Autodesk Inventor part; units mm, degrees
ref_plane "YZ Plane" through (0, 0, 0) normal (1, 0, 0) x (0, 1, 0)
ref_plane "XZ Plane" through (0, 0, 0) normal (0, 1, 0) x (-1, 0, 0)
ref_plane "XY Plane" through (0, 0, 0) normal (0, 0, 1) x (1, 0, 0)
sketch "Sketch1" plane through (0, 0, 0) normal (0, 0, 1) x (1, 0, 0)
  line L0 (0, 0) -> (12.7, 0)
  line L1 (12.7, 0) -> (12.7, 12.7)
  line L2 (12.7, 12.7) -> (0, 12.7)
  line L3 (0, 12.7) -> (0, 0)
  circle A0 centre (6.35, 6.35) radius 5.08
  dimension "d0" = 12.7
  dimension "d1" = 12.7
  dimension "d2" = 10.16
extrude "Extrusion1" add sketch "Sketch1" along normal blind 3.175
extrude "Extrusion2" add sketch "Sketch1" along normal blind 12.7 contours A0
sketch "Sketch2" plane through (6.35, 6.35, 12.7) normal (0, 0, 1) x (1, 0, 0)
  circle A0 centre (0, 0) radius 2.2451
  point P0 (-6.35, -6.35)
extrude "Extrusion3" cut sketch "Sketch2" against normal blind 25.4
properties part number "TestPart1"
The listing builds one solid part. Answer for the finished solid, in the listing's coordinates (mm). A direction names the side the tool comes from. Give positions to 0.01 mm unless a question says otherwise; leave off trailing zeros. Order: outer loops, then holes, each group sorted by start corner. A loop starts at its lowest first (then second) coordinate and runs counter-clockwise, first axis right, second up. Notation, with made-up numbers: (21.25, 8.5) - (66.25, 8.5) arc R8 cw to (66.25, 12.5) - close; hole circle Ø5 at (79.5, 88.5). An arc over 180 degrees is marked (long way). Answer as CSV lines item,"result".
Q1. A cutting plane is placed at C-C, the plane z = 2.5. Determine the outline of the cut face in (x, y), and give its area (3 significant figures).
Answer key:
outline,"(0, 0) - (12.7, 0) - (12.7, 12.7) - (0, 12.7) - close; hole circle Ø4.49 at (6.35, 6.35)"
area,"145 mm^2"
Q2. A cutting plane is placed at A-A, the plane y = 6.35. Determine the outline of the cut face in (x, z) (3 decimals).
Answer key:
outline,"(0, 0) - (4.105, 0) - (4.105, 12.7) - (1.27, 12.7) - (1.27, 3.175) - (0, 3.175) - close; (8.595, 0) - (12.7, 0) - (12.7, 3.175) - (11.43, 3.175) - (11.43, 12.7) - (8.595, 12.7) - close"
Q3. Straight lines are drawn through the part: L1, parallel to Y at x = 6.35, z = 9; L2, parallel to Z at x = 1, y = 8.5 (3 decimals); L3, parallel to X at y = 7, z = 11. For each, find the intervals that lie inside material, in ascending order.
Answer key:
L1,"y = 1.27 to 4.1, 8.6 to 11.43"
L2,"z = 0 to 3.175"
L3,"x = 1.31 to 4.2, 8.5 to 11.39"
Q4. Which of the six approach directions +Z, -Z, +X, -X, +Y, -Y give full straight-line access (tool end or side, diameter ignored) to faces 5 (the face through (3, 11, 3.175)), 6 (the face through (6, 0, 2))?
Answer key:
face 5,"+Z"
face 6,"+Z, -Z, +X, -X, -Y"
Q5. Each of these flat-tipped pins is pushed along its axis until it touches: pin 1 Ø1.5 at (x, z) = (3.5, 6.5) entering from -Y; pin 2 Ø4 at (y, z) = (9, 9.5) entering from +X; pin 3 Ø4 at (y, z) = (10.5, 5.5) entering from -X. Where does it stop, or does it pass through?
Answer key:
pin 1,"stops at y = 1.72"
pin 2,"stops at x = 11.39"
pin 3,"stops at x = 1.75"
Q6. Determine the mould class of faces 1 (the face through (9, 6, 0)), 2 (the face through (7.56, 8.24, 6.44)), 3 (the face through (0, 6, 2)), 4 (the face through (8.69, 10.86, 7.87)) for opening direction X: pulls with the +X half, pulls with the -X half, needs draft (parallel to the pull), parting line crosses it, or undercut.
Answer key:
face 1,"needs draft"
face 2,"undercut"
face 3,"pulls with the -X half"
face 4,"parting line crosses it"
Q7. A cutting plane is placed at D-D, the plane y = 11. Determine the outline of the cut face in (x, z) (3 decimals).
Answer key:
outline,"(0, 0) - (12.7, 0) - (12.7, 3.175) - (8.395, 3.175) - (8.395, 12.7) - (4.305, 12.7) - (4.305, 3.175) - (0, 3.175) - close"
